```python
from build123d import *

# Parameters (mm, degrees)
BOSS_EXTRUDE2_DEPTH = 3.5
SKETCH4_R           = 1
CUT_EXTRUDE1_DEPTH  = 8.797595783
SKETCH5_W           = 5
SKETCH5_H           = 3.95
CUT_EXTRUDE2_DEPTH  = 6
SKETCH7_R           = 1
BOSS_EXTRUDE3_DEPTH = 1
SKETCH8_R           = 0.8
CUT_EXTRUDE3_DEPTH  = 2


with BuildPart() as part:
    # Sketch1 → Boss-Extrude2 (new, symmetric)
    with BuildSketch(Plane.XY):
        with BuildLine():
            Line((-1.25, 0), (-1.25, 3.2))
            Line((-1.25, 3.2), (1.25, 3.2))
            Line((1.25, 3.2), (1.25, 0))
            ThreePointArc((1.25, 0), (0, -1.25), (-1.25, 0))
        make_face()
    extrude(amount=BOSS_EXTRUDE2_DEPTH, both=True)

    # Sketch4 → Cut-Extrude1 (cut, through all)
    with BuildSketch(Plane.XY.offset(3.5)):
        Circle(SKETCH4_R)
    extrude(amount=-CUT_EXTRUDE1_DEPTH, mode=Mode.SUBTRACT)

    # Sketch5 → Cut-Extrude2 (cut)
    with BuildSketch(Plane.ZY.offset(1.25)):
        with Locations((0, 0.725)):
            Rectangle(SKETCH5_W, SKETCH5_H)
    extrude(amount=-CUT_EXTRUDE2_DEPTH, mode=Mode.SUBTRACT)

    # Sketch7 → Boss-Extrude3 (add)
    with BuildSketch(Plane(origin=(0, 3.2, 0), x_dir=(1, 0, 0), z_dir=(0, 1, 0))):
        with Locations(Location((0, 0, 0), (0, 0, 270))):
            Circle(SKETCH7_R)
    extrude(amount=BOSS_EXTRUDE3_DEPTH)

    # Sketch8 → Cut-Extrude3 (cut)
    with BuildSketch(Plane(origin=(0, 4.2, 0), x_dir=(1, 0, 0), z_dir=(0, 1, 0))):
        with Locations(Location((0, 0, 0), (0, 0, 270))):
            Circle(SKETCH8_R)
    extrude(amount=-CUT_EXTRUDE3_DEPTH, mode=Mode.SUBTRACT)


solid = part.part
```
Can you work these out from the model? Positions are in its coordinate system, mm. A direction names the side the tool comes from. Coordinates: 2 decimals unless noted, no trailing zeros. Loops run counter-clockwise (first coordinate to the right, second up) from the corner with the lowest first, then second, coordinate; pieces in that order, holes last. Notation, with made-up numbers: (-20, 6.25) -> (9, 6.25) arc R31 ccw to (9, 40.25) -> close; hole circle Ø9 at (14, 56). An arc over 180 degrees is marked (long way). Answer as a JSON object with one key per item and string values.
1) Imagine slicing it at B-B (z = 0). Please give me the cut outline in (x, y).
Results:
{"outline": "(-1.25, 2.7) -> (-0.8, 2.7) -> (-0.8, 4.2) -> (-1, 4.2) -> (-1, 3.2) -> (-1.25, 3.2) -> close; (0.8, 2.7) -> (1.25, 2.7) -> (1.25, 3.2) -> (1, 3.2) -> (1, 4.2) -> (0.8, 4.2) -> close"}
2) If I drill on line 1 (X direction, y = 3.6, z = 0); line 2 (Y direction, x = 0, z = -3.2); line 3 (Z direction, x = 0.45, y = 1.1), over which ranges is the centre line in solid material (lowest first)?
Results:
{"line 1": "x = -1 to -0.8, 0.8 to 1", "line 2": "y = -1.25 to -1, 1 to 3.2", "line 3": "z = -3.5 to -2.5, 2.5 to 3.5"}
3) Imagine slicing it at A-A (x = 0). Please give me the cut outline in (y, z).
Results:
{"outline": "(-1.25, -3.5) -> (-1, -3.5) -> (-1, -2.5) -> (-1.25, -2.5) -> close; (-1.25, 2.5) -> (-1, 2.5) -> (-1, 3.5) -> (-1.25, 3.5) -> close; (1, -3.5) -> (3.2, -3.5) -> (3.2, -1) -> (4.2, -1) -> (4.2, -0.8) -> (2.7, -0.8) -> (2.7, -2.5) -> (1, -2.5) -> close; (1, 2.5) -> (2.7, 2.5) -> (2.7, 0.8) -> (4.2, 0.8) -> (4.2, 1) -> (3.2, 1) -> (3.2, 3.5) -> (1, 3.5) -> close"}
4) Imagine slicing it at C-C (y = 1.2). Please give me the cut outline in (x, z).
Results:
{"outline": "(-1.25, -3.5) -> (1.25, -3.5) -> (1.25, -2.5) -> (-1.25, -2.5) -> close; (-1.25, 2.5) -> (1.25, 2.5) -> (1.25, 3.5) -> (-1.25, 3.5) -> close"}
5) For faces 1 (the face through (-1, 2.7, -1)), 2 (the face through (0, 2, 3.5)), 3 (the face through (-1, 4, 0)), which set-ups out of +Z, -Z, +X, -X, +Y, -Y let a thin tool reach every point of the face, with its end or its side?
Results:
{"face 1": "+X, -X, -Y", "face 2": "+Z, +X, -X, +Y, -Y", "face 3": "+Y"}
6) Imagine slicing it at D-D (z = 3). Please give me the cut outline in (x, y), then the cut area to 3 significant figures.
Results:
{"outline": "(-1.25, 0) arc R1.25 ccw to (1.25, 0) -> (1.25, 3.2) -> (-1.25, 3.2) -> close; hole circle Ø2 at (0, 0)", "area": "7.31 mm^2"}
7) Thinking about a two-plate mould opening in Y: for faces 4 (the face through (-1, 3.2, 1)), 5 (the face through (0, -1, 3)), 6 (the face through (-1.25, 3, 0)), which applies, pulls with the +Y half, pulls with the -Y half, needs draft (parallel to the pull), parting line crosses it, or undercut?
Results:
{"face 4": "pulls with the +Y half", "face 5": "undercut", "face 6": "needs draft"}
8) For P1, Ø1.5, axis at y = 3.5, z = -1, coming from the +X side, with a flat end and sliding along its axis, tell me the tip position at first contact or that it passes through.
Results:
{"P1": "stops at x = 1.25"}
